from build123d import *

# Parameters (mm, degrees)
SKETCH1_R               = 12.065
BOSS_EXTRUDE1_DEPTH     = 10.795
SKETCH5_W               = 38.1
SKETCH5_H               = 21.59
BOSS_EXTRUDE2_DEPTH     = 101.6
CUT_EXTRUDE1_REACH      = 261.255
SKETCH6_R               = 3.175
SKETCH4_W               = 12.7
SKETCH4_H               = 21.59
BOSS_EXTRUDE3_DEPTH     = 50.8
CUT_EXTRUDE2_DEPTH      = 210.73176208
CUT_EXTRUDE2_DEPTH_BACK = 210.73176208
SKETCH6_2_R             = 3.175
CUT_EXTRUDE3_DEPTH      = 214.164307578
CUT_EXTRUDE3_DEPTH_BACK = 214.164307578


with BuildPart() as part:
    # Sketch1 → Boss-Extrude1 (new, symmetric)
    with BuildSketch(Plane(origin=(0, 0, 0), x_dir=(1, 0, 0), z_dir=(0, 1, 0))):
        with BuildLine():
            Line((-31.75, 152.4), (31.75, 152.4))
            ThreePointArc((31.75, 152.4), (21.755106695, 76.491146914), (18.415, 0))
            ThreePointArc((18.415, 0), (0, -18.415), (-18.415, 0))
            ThreePointArc((-18.415, 0), (-21.755106695, 76.491146914), (-31.75, 152.4))
        make_face()
        with Locations(Location((0, 0, 0), (0, 0, 270))):
            Circle(SKETCH1_R, mode=Mode.SUBTRACT)
    extrude(amount=BOSS_EXTRUDE1_DEPTH, both=True)

    # Sketch5 → Boss-Extrude2 (add)
    with BuildSketch(Plane(origin=(0, 0, -152.4), x_dir=(-1, 0, 0), z_dir=(0, 0, -1))):
        Rectangle(SKETCH5_W, SKETCH5_H)
    extrude(amount=BOSS_EXTRUDE2_DEPTH)

    # Sketch6 → Cut-Extrude1 (cut, up to next)
    with BuildSketch(Plane(origin=(19.05, 0, 0), x_dir=(0, 0, -1), z_dir=(1, 0, 0)), mode=Mode.PRIVATE) as cut_extrude1_sk1:
        Polygon((152.4, -10.795), (154.288880246, 10.795), (254, 10.795), (254, -10.795), align=None)
        with Locations((185.094440123, 0)):
            Circle(SKETCH6_R, mode=Mode.SUBTRACT)
    cut_extrude1_tool1 = extrude(cut_extrude1_sk1.sketch, amount=-CUT_EXTRUDE1_REACH, mode=Mode.PRIVATE) & part.part
    add(cut_extrude1_tool1.solids().sort_by_distance((19.05, -0.034262, -203.945458))[0], mode=Mode.SUBTRACT)


with BuildPart() as cut_extrude1_piece_1:
    # of the separate pieces the step leaves, piece 1, a body of its own (cut_extrude1_pieces)
    add(part.part.solids().sort_by_distance((-31.75, -10.795, -152.4))[0])

    # Sketch4 → Boss-Extrude3 (add)
    with BuildSketch(Plane(origin=(0, 0, -152.4), x_dir=(-1, 0, 0), z_dir=(0, 0, -1))):
        with Locations((-25.4, 0)):
            Rectangle(SKETCH4_W, SKETCH4_H)
        with Locations((25.4, 0)):
            Rectangle(SKETCH4_W, SKETCH4_H)
    extrude(amount=BOSS_EXTRUDE3_DEPTH)


with BuildPart() as cut_extrude1_piece_2:
    # of the separate pieces the step leaves, piece 2, a body of its own (cut_extrude1_pieces)
    add(part.part.solids().sort_by_distance((-19.05, 0, -188.269440123))[0])


with BuildPart() as cut_extrude2_tool:
    # Sketch6_2 → Cut-Extrude2 (new, two sides: drawn at the far end of the back side and taken through both)
    with BuildSketch(Plane(origin=(19.05, 0, 0), x_dir=(0, 0, -1), z_dir=(1, 0, 0)).offset(-CUT_EXTRUDE2_DEPTH_BACK)):
        with Locations((185.094440123, 0)):
            Circle(SKETCH6_2_R)
    extrude(amount=CUT_EXTRUDE2_DEPTH + CUT_EXTRUDE2_DEPTH_BACK)


with BuildPart() as cut_extrude1_piece_1_1:
    add(cut_extrude1_piece_1.part)

    # Cut-Extrude2: cut by cut_extrude2_tool
    add(cut_extrude2_tool.part, mode=Mode.SUBTRACT)

    # Sketch7 → Cut-Extrude3 (cut, two sides: drawn at the far end of the back side and taken through both)
    with BuildSketch(Plane(origin=(31.75, 0, 0), x_dir=(0, 0, -1), z_dir=(1, 0, 0)).offset(-CUT_EXTRUDE3_DEPTH_BACK)):
        with BuildLine():
            Line((203.2, 10.795), (185.094440123, 10.795))
            ThreePointArc((185.094440123, 10.795), (192.727657826, 7.633217703), (195.889440123, 0))
            ThreePointArc((195.889440123, 0), (192.727657826, -7.633217703), (185.094440123, -10.795))
            Line((185.094440123, -10.795), (203.2, -10.795))
            Line((203.2, -10.795), (203.2, 10.795))
        make_face()
    extrude(amount=CUT_EXTRUDE3_DEPTH + CUT_EXTRUDE3_DEPTH_BACK, mode=Mode.SUBTRACT)


with BuildPart() as cut_extrude1_piece_2_1:
    add(cut_extrude1_piece_2.part)

    # Cut-Extrude2: cut by cut_extrude2_tool
    add(cut_extrude2_tool.part, mode=Mode.SUBTRACT)


solid = cut_extrude1_piece_1_1.part
Input: part model. Units: mm. Frame: model coordinates. Coordinates: 2 decimals unless noted, no trailing zeros. Loops run counter-clockwise (first coordinate to the right, second up) from the corner with the lowest first, then second, coordinate; pieces in that order, holes last.
Q1. Cut plane C-C (x = 27). Output: boundary loops of the cut face in (y, z) (3 decimals).
Q2. Contact query for a flat-ended pin moving along its axis: pin 1 (8 mm diameter, centred on y = 0.5, z = -71.5, fed in from +X). Output: stop coordinate, or through.
Q3. Draft query along Z for faces 1 (the face through (0, -10.795, -105)), 2 (the face through (0.27, -0.15, -153.33)), 3 (the face through (-25.489, 0.14, -181.923)). Return one class per face: +Z half, -Z half, draft (parallel to the pull), parting line (faces both ways), or undercut.
Q4. Cut plane B-B (y = -5). Output: boundary loops of the cut face in (x, z) (3 decimals), then the cut area to 3 significant figures.
Q5. Material intervals for line 1 (X direction, y = -2.75, z = -170); line 2 (X direction, y = 3.75, z = 0.5); line 3 (Z direction, x = -11, y = 0.75), sorted ascending.
Q6. Cut plane D-D (x = -6.5). Output: boundary loops of the cut face in (y, z) (3 decimals), then the cut area to 3 significant figures.
Q7. Cut plane A-A (x = 3). Output: boundary loops of the cut face in (y, z) (3 decimals), then the cut area to 3 significant figures.
Working result:
1. outline: (-10.795, -185.094) arc R10.795 ccw to (10.795, -185.094) - (10.795, -122.448) - (-10.795, -122.448) - close; hole circle Ø6.35 at (0, -185.094)
2. pin 1: stops at x = 21.67
3. face 1: draft
3. face 2: -Z half
3. face 3: undercut
4. outline: (-31.75, -194.662) - (-19.05, -194.662) - (-19.05, -152.907) - (19.05, -152.907) - (19.05, -194.662) - (31.75, -194.662) - (31.75, -152.4) arc R877.525 cw to (18.415, 0) arc R18.415 ccw to (-18.415, 0) arc R877.525 cw to (-31.75, -152.4) - close; hole circle Ø24.13 at (0, 0)
4. area: 8,130 mm2
5. line 1: x = -31.75 to -19.05, 19.05 to 31.75
5. line 2: x = -18.41 to -12.05, 12.05 to 18.41
5. line 3: z = -153.41 to -4.96, 4.96 to 14.77
6. outline: (-10.795, -152.4) - (10.795, -154.289) - (10.795, -10.164) - (-10.795, -10.164) - close; (-10.795, 10.164) - (10.795, 10.164) - (10.795, 17.23) - (-10.795, 17.23) - close
6. area: 3,240 mm2
7. outline: (-10.795, -152.4) - (10.795, -154.289) - (10.795, -11.686) - (-10.795, -11.686) - close; (-10.795, 11.686) - (10.795, 11.686) - (10.795, 18.169) - (-10.795, 18.169) - close
7. area: 3,200 mm2
